from build123d import *

# Parameters (mm, degrees)
BOSS_EXTRUDE1_DEPTH  = 10
FILLET2_R            = 1
FILLET2_OF_MIRROR1_R = 1
CUT_EXTRUDE1_DEPTH   = 81.635062113
FILLET3_R            = 1
SKETCH5_R            = 2.5
BOSS_EXTRUDE2_DEPTH  = 10
FILLET1_R            = 0.5
CUT_EXTRUDE2_DEPTH   = 10


with BuildPart() as part:
    # Sketch2 → Boss-Extrude1 (new body)
    with BuildSketch(Plane(origin=(0, 0, 0), x_dir=(1, 0, 0), z_dir=(0, 1, 0))):
        Polygon((-19.893799085, 77.5), (0, 77.5), (0, 75.5), (-2.625, 75.5), (-2.625, 73), (-2.625, 63), (-2.625, 60.5), (0, 60.5), (0, 60.375), (0, 2.5), (-2.625, 2.5), (-2.625, 0), (-2.625, -10), (-2.625, -12.5), (0, -12.5), (0, -14.5), (-19.893799085, -14.5), align=None)
    boss_extrude1 = extrude(amount=BOSS_EXTRUDE1_DEPTH)

    # Fillet2
    fillet2_edges = [part.edges().sort_by_distance(p)[0] for p in [
        (-2.625, 5, 12.5),
        (-2.625, 5, -2.5),
        (-2.625, 5, -60.5),
        (-2.625, 5, -75.5),
    ]]
    fillet(fillet2_edges, radius=FILLET2_R)

    # Mirror1: Boss-Extrude1 across Right Plane
    add(boss_extrude1.mirror(Plane(origin=(0, 0, 0), x_dir=(0, 0, -1), z_dir=(1, 0, 0))))

    # Fillet2 of Mirror1
    fillet2_of_mirror1_edges = [part.edges().sort_by_distance(p)[0] for p in [
        (2.625, 5, 12.5),
        (2.625, 5, -2.5),
        (2.625, 5, -60.5),
        (2.625, 5, -75.5),
    ]]
    fillet(fillet2_of_mirror1_edges, radius=FILLET2_OF_MIRROR1_R)

    # Sketch4 → Cut-Extrude1 (cut, through all)
    with BuildSketch(Plane(origin=(0, 0, 0), x_dir=(1, 0, 0), z_dir=(0, 1, 0))):
        Polygon((-14.625, 15), (-14.625, 5), (-14.625, 2.5), (-12, 2.5), (-9.375, 2.5), (-9.375, 5), (-9.375, 15), (-9.375, 17.5), (-12, 17.5), (-14.625, 17.5), align=None)
        Polygon((9.375, 58), (9.375, 48), (9.375, 45.5), (12, 45.5), (14.625, 45.5), (14.625, 48), (14.625, 58), (14.625, 60.5), (12, 60.5), (9.375, 60.5), align=None)
    extrude(amount=CUT_EXTRUDE1_DEPTH, mode=Mode.SUBTRACT)

    # Fillet3
    fillet3_edges = [part.edges().sort_by_distance(p)[0] for p in [
        (-14.625, 5, -17.5),
        (-14.625, 5, -2.5),
        (-9.375, 5, -2.5),
        (-9.375, 5, -17.5),
        (14.625, 5, -60.5),
        (9.375, 5, -60.5),
        (9.375, 5, -45.5),
        (14.625, 5, -45.5),
    ]]
    fillet(fillet3_edges, radius=FILLET3_R)

    # Sketch5 → Boss-Extrude2 (add)
    with BuildSketch(Plane(origin=(0, 10, 0), x_dir=(1, 0, 0), z_dir=(0, 1, 0))):
        with Locations(Location((0, 31.5, 0), (0, 0, 90))):
            Circle(SKETCH5_R)
    extrude(amount=BOSS_EXTRUDE2_DEPTH)

    # Fillet1
    fillet1_edges = [part.edges().sort_by_distance(p)[0] for p in [
        (0, 10, -29),
    ]]
    fillet(fillet1_edges, radius=FILLET1_R)

    # Sketch6 → Cut-Extrude2 (cut)
    with BuildSketch(Plane(origin=(0, 10, 0), x_dir=(1, 0, 0), z_dir=(0, 1, 0))):
        Polygon((19.893799085, 77.5), (19.893799085, 67.609192382), (6.623799085, 67.609192382), (6.623799085, 43.5), (-6.625, 43.5), (-19.893799085, 43.5), (-19.893799085, 77.5), (-6.625, 77.5), align=None)
    extrude(amount=-CUT_EXTRUDE2_DEPTH, mode=Mode.SUBTRACT)


solid = part.part
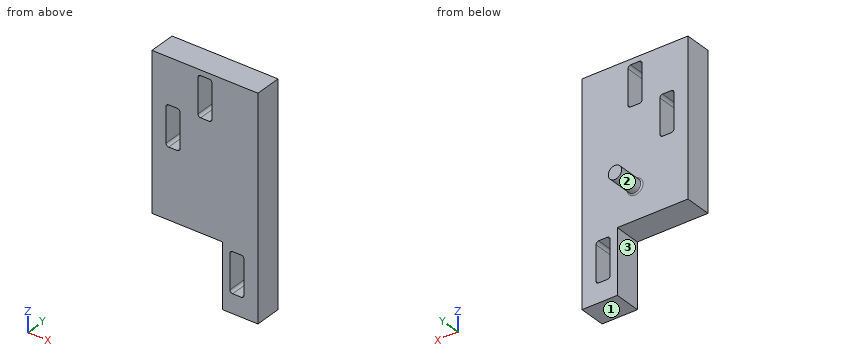
The model under review builds one solid part; all positions refer to its coordinate system, in mm. Face numbers are marked on the shaded views. A direction names the side the tool comes from. Give positions to 0.01 mm unless a question says otherwise; leave off trailing zeros. Loops run counter-clockwise (first coordinate to the right, second up) from the corner with the lowest first, then second, coordinate; pieces in that order, holes last. Notation, with made-up numbers: (64.25, 34) -> (113.25, 34) arc R18 ccw to (113.25, 55) -> close; hole circle Ø1 at (18.25, 58). An arc over 180 degrees is marked (long way). Put each result on its own line as item: value. Start each with the question number.
1. Wall thickness on probe 1 along X at (y, z) = (6.75, -10) (3 decimals); probe 2 along X at (y, z) = (1, -55) (3 decimals); probe 3 along Z at (x, y) = (11, 9): over which ranges is each line inside the solid? List them lowest first.
2. We need section A-A on x = -12. State the section outline as (y, z) points, then the cut area to 3 significant figures.
3. Clearance check with flat-ended pins moving along their axes: P1, Ø8, axis at y = 6, z = -55.5, coming from the -X side; P2, Ø1, axis at x = 3, z = -22.5, coming from the -Y side; P3, Ø5, axis at x = -6.5, y = 4.5, coming from the -Z side; P4, Ø5, axis at x = -5.5, z = -17.5, coming from the +Y side. State where each tip first meets the part, or that it passes through.
4. For the marked faces 1, 2 and 3, list the 3-axis set-ups (+Z, -Z, +X, -X, +Y, -Y) from which the entire face can be reached by the end or side of a thin tool; tool diameter is ignored.
5. We need section D-D on z = -31.5. State the section outline as (x, y) points, then the cut area to 3 significant figures.
6. We need section B-B on z = 0.5. State the section outline as (x, y) points (3 decimals), then the cut area to 3 significant figures.
7. We need section C-C on y = 4. State how many separate pieces and enclosed holes the cut face has, then the cut area to 3 significant figures.
Determined:
1. probe 1: -19.894 to -14.625, -9.375 to 19.894
1. probe 2: 6.624 to 9.375, 14.625 to 19.894
1. probe 3: -67.61 to -60.5, -45.5 to 14.5
2. outline: (0, -43.5) -> (10, -43.5) -> (10, -17.5) -> (0, -17.5) -> close; (0, -2.5) -> (10, -2.5) -> (10, 14.5) -> (0, 14.5) -> close
2. area: 430 mm^2
3. P1: x = 6.62
3. P2: y = 0
3. P3: z = -43.5
3. P4: y = 10
4. face 1: -Z, +X, -X, +Y, -Y
4. face 2: +Y
4. face 3: -Z, -X, +Y, -Y
5. outline: (-19.89, 0) -> (19.89, 0) -> (19.89, 10) -> (3, 10) arc R0.5 cw to (2.5, 10.5) -> (2.5, 20) -> (-2.5, 20) -> (-2.5, 10.5) arc R0.5 cw to (-3, 10) -> (-19.89, 10) -> close
5. area: 448 mm^2
6. outline: (-19.894, 0) -> (-2.625, 0) -> (-2.625, 10) -> (-19.894, 10) -> close; (2.625, 0) -> (19.894, 0) -> (19.894, 10) -> (2.625, 10) -> close
6. area: 345 mm^2
7. separate pieces: 1
7. enclosed holes: 3
7. area: 2,390 mm^2
